from build123d import *

# Parameters (mm, degrees)
SKETCH1_W            = 388.7
SKETCH1_H            = 435.95
SKETCH1_W_2          = 45.6
SKETCH1_H_2          = 430.25
BOSS_EXTRUDE1_DEPTH  = 189
BOSS_EXTRUDE2_START  = -433.45
SKETCH2_W            = 388.7
SKETCH2_H            = 3.2
BOSS_EXTRUDE2_DEPTH  = 430.25
CUT_EXTRUDE1_DEPTH   = 25
BOSS_EXTRUDE4_DEPTH  = 3.2
BOSS_EXTRUDE5_DEPTH  = 3.2
BOSS_EXTRUDE6_REACH  = 791.664
CUT_EXTRUDE2_REACH   = 793.231
SKETCH11_W           = 52.59
SKETCH11_H           = 168.019571709
BOSS_EXTRUDE7_DEPTH  = 3.2
BOSS_EXTRUDE8_DEPTH  = 3.2
SKETCH14_W           = 388.7
SKETCH14_H           = 3.2
BOSS_EXTRUDE9_DEPTH  = 40
SKETCH15_W           = 388.7
SKETCH15_H           = 3.2
BOSS_EXTRUDE10_DEPTH = 40
SKETCH16_W           = 693.36
SKETCH16_H           = 3.2
BOSS_EXTRUDE11_DEPTH = 43.15
SKETCH17_W           = 693.36
SKETCH17_H           = 3.2
BOSS_EXTRUDE12_DEPTH = 43.15
BOSS_EXTRUDE13_DEPTH = 388.7


with BuildPart() as part:
    # Sketch1 → Boss-Extrude1 (new body)
    with BuildSketch(Plane(origin=(0, 0, 0), x_dir=(1, 0, 0), z_dir=(0, 1, 0))):
        with Locations((191.15, 214.775)):
            Rectangle(SKETCH1_W, SKETCH1_H)
        with Locations((22.8, 215.125)):
            Rectangle(SKETCH1_W_2, SKETCH1_H_2, mode=Mode.SUBTRACT)
        with Locations((359.5, 215.125)):
            Rectangle(SKETCH1_W_2, SKETCH1_H_2, mode=Mode.SUBTRACT)
        with Locations((70.9, 215.125)):
            Rectangle(SKETCH1_W_2, SKETCH1_H_2, mode=Mode.SUBTRACT)
        with Locations((119, 215.125)):
            Rectangle(SKETCH1_W_2, SKETCH1_H_2, mode=Mode.SUBTRACT)
        with Locations((167.1, 215.125)):
            Rectangle(SKETCH1_W_2, SKETCH1_H_2, mode=Mode.SUBTRACT)
        with Locations((215.2, 215.125)):
            Rectangle(SKETCH1_W_2, SKETCH1_H_2, mode=Mode.SUBTRACT)
        with Locations((263.3, 215.125)):
            Rectangle(SKETCH1_W_2, SKETCH1_H_2, mode=Mode.SUBTRACT)
        with Locations((311.4, 215.125)):
            Rectangle(SKETCH1_W_2, SKETCH1_H_2, mode=Mode.SUBTRACT)
    extrude(amount=BOSS_EXTRUDE1_DEPTH)

    # Sketch2 → Boss-Extrude2 (add)
    with BuildSketch(Plane.XY.offset(3.2).offset(BOSS_EXTRUDE2_START)):
        with Locations((191.15, 1.6)):
            Rectangle(SKETCH2_W, SKETCH2_H)
    extrude(amount=BOSS_EXTRUDE2_DEPTH)

    # Sketch3 → Cut-Extrude1 (cut)
    with BuildSketch(Plane(origin=(0, 189, 0), x_dir=(1, 0, 0), z_dir=(0, 1, 0))):
        Polygon((0, 430.25), (0, 432.75), (382.3, 432.75), (382.3, 430.25), (336.7, 430.25), (336.7, 0), (334.2, 0), (334.2, 430.25), (288.6, 430.25), (288.6, 0), (286.1, 0), (286.1, 430.25), (240.5, 430.25), (240.5, 0), (238, 0), (238, 430.25), (192.4, 430.25), (192.4, 0), (189.9, 0), (189.9, 430.25), (144.3, 430.25), (144.3, 0), (141.8, 0), (141.8, 430.25), (96.2, 430.25), (96.2, 0), (93.7, 0), (93.7, 430.25), (48.1, 430.25), (48.1, 0), (45.6, 0), (45.6, 430.25), align=None)
    extrude(amount=-CUT_EXTRUDE1_DEPTH, mode=Mode.SUBTRACT)

    # Sketch4 → Boss-Extrude4 (add)
    with BuildSketch(Plane(origin=(385.5, 0, 0), x_dir=(0, 0, -1), z_dir=(1, 0, 0))):
        Polygon((432.75, 189), (662.75, 0), (432.75, 0), align=None)
    extrude(amount=-BOSS_EXTRUDE4_DEPTH)

    # Sketch7 → Boss-Extrude5 (add)
    with BuildSketch(Plane.ZY.offset(3.2)):
        Polygon((-432.75, 164), (-432.75, 189), (-662.75, 0), (-432.75, 0), align=None)
    extrude(amount=-BOSS_EXTRUDE5_DEPTH)

    # Sketch9 → Boss-Extrude6 (add, up to next)
    with BuildSketch(Plane(origin=(0, 0, 0), x_dir=(0, 0, -1), z_dir=(1, 0, 0)), mode=Mode.PRIVATE) as boss_extrude6_sk1:
        Polygon((662.75, 0), (658.855820106, 3.2), (432.75, 3.2), (432.75, 0), align=None)
    boss_extrude6_tool1 = extrude(boss_extrude6_sk1.sketch, amount=BOSS_EXTRUDE6_REACH, mode=Mode.PRIVATE) - part.part
    add(boss_extrude6_tool1.solids().sort_by_distance((0, 1.595446, -546.779226))[0])

    # Sketch11 → Cut-Extrude2 (cut, up to next)
    with BuildSketch(Plane(origin=(385.5, 0, 0), x_dir=(0, 0, -1), z_dir=(1, 0, 0)), mode=Mode.PRIVATE) as cut_extrude2_sk1:
        with Locations((636.455, 84.009785855)):
            Rectangle(SKETCH11_W, SKETCH11_H)
    cut_extrude2_tool1 = extrude(cut_extrude2_sk1.sketch, amount=-CUT_EXTRUDE2_REACH, mode=Mode.PRIVATE) & part.part
    add(cut_extrude2_tool1.solids().sort_by_distance((385.5, 84.009786, -636.455))[0], mode=Mode.SUBTRACT)

    # Sketch12 → Boss-Extrude7 (add)
    with BuildSketch(Plane(origin=(385.5, 0, 0), x_dir=(0, 0, -1), z_dir=(1, 0, 0))):
        Polygon((456.376412276, 189), (610.16, 62.630008348), (610.16, 43.21526087), (432.75, 189), align=None)
    extrude(amount=-BOSS_EXTRUDE7_DEPTH)

    # Sketch13 → Boss-Extrude8 (add)
    with BuildSketch(Plane.ZY.offset(3.2)):
        Polygon((-610.16, 62.630008348), (-610.16, 43.21526087), (-432.75, 189), (-456.376412276, 189), align=None)
    extrude(amount=-BOSS_EXTRUDE8_DEPTH)

    # Sketch14 → Boss-Extrude9 (add)
    with BuildSketch(Plane(origin=(0, 0, -610.16), x_dir=(-1, 0, 0), z_dir=(0, 0, -1))):
        with Locations((-191.15, 1.6)):
            Rectangle(SKETCH14_W, SKETCH14_H)
    extrude(amount=BOSS_EXTRUDE9_DEPTH)

    # Sketch15 → Boss-Extrude10 (add)
    with BuildSketch(Plane.XY.offset(3.2)):
        with Locations((191.15, 1.6)):
            Rectangle(SKETCH15_W, SKETCH15_H)
    extrude(amount=BOSS_EXTRUDE10_DEPTH)

    # Sketch16 → Boss-Extrude11 (add)
    with BuildSketch(Plane(origin=(385.5, 0, 0), x_dir=(0, 0, -1), z_dir=(1, 0, 0))):
        with Locations((303.48, 1.6)):
            Rectangle(SKETCH16_W, SKETCH16_H)
    extrude(amount=BOSS_EXTRUDE11_DEPTH)

    # Sketch17 → Boss-Extrude12 (add)
    with BuildSketch(Plane.ZY.offset(3.2)):
        with Locations((-303.48, 1.6)):
            Rectangle(SKETCH17_W, SKETCH17_H)
    extrude(amount=BOSS_EXTRUDE12_DEPTH)

    # Sketch18 → Boss-Extrude13 (add)
    with BuildSketch(Plane.ZY.offset(3.2)):
        Polygon((-457.200187026, 191.3), (3.2, 191.3), (3.2, 189), (-456.376412276, 189), (-610.16, 62.630008348), (-610.16, 3.2), (-612.46, 3.2), (-612.46, 63.716936295), align=None)
    extrude(amount=-BOSS_EXTRUDE13_DEPTH)


solid = part.part
For this review, take the finished solid that the model builds, in its own axes (mm). A direction names the side the tool comes from. Give positions to 0.01 mm unless a question says otherwise; leave off trailing zeros. Loops run counter-clockwise (first coordinate to the right, second up) from the corner with the lowest first, then second, coordinate; pieces in that order, holes last.
Item 1: Tool access review of faces 1 (the flat face through (-3.2, 99, -300)), 2 (the flat face through (288.6, 82, -212)): name each direction out of +Z, -Z, +X, -X, +Y, -Y from which nothing blocks a thin tool from reaching the whole face with its end or side.
Item 2: For line 1 along Z through (x, y) = (90, 17); line 2 along Y through (x, z) = (82, -298.5); line 3 along Z through (x, y) = (326, 132.5), list the stretches that pass through material, from the lowest coordinate up.
Item 3: Draft analysis for pull direction X (two halves, no side actions). For faces 3 (the flat face through (385.5, 99, -300)), 4 (the flat face through (188, 99, 3.2)), 5 (the flat face through (188.47, 126.7, -532.19)), 6 (the flat face through (359, 82, -430.25)), state which applies: +X half, -X half, draft (parallel to the pull), parting line (faces both ways), or undercut.
Item 4: Take a section at B-B, the plane z = -531.5. State the section outline as (x, y) points, and give its area (3 significant figures).
Item 5: Take a section at C-C, the plane y = 31. Give the number of separate pieces and of enclosed holes in the cut face, and give its area (3 significant figures).
Item 6: Insertion check: pin 1 (1 mm diameter, centred on y = 67.5, z = -159.5, fed in from -X); pin 2 (2 mm diameter, centred on x = 285.5, y = 30, fed in from +Z); pin 3 (6 mm diameter, centred on y = 132, z = -139, fed in from +X). Each pin has a flat end and moves straight along its axis. Give the tip position at first contact, or say it passes through.
Item 7: Take a section at A-A, the plane x = 173. State the section outline as (y, z) points, and give its area (3 significant figures).
Calculated:
1. face 1: +Z, -Z, -X, +Y
1. face 2: none
2. line 1: z = -612.46 to -610.16, -432.75 to -430.25, 0 to 3.2
2. line 2: y = 0 to 3.2, 189 to 191.3
2. line 3: z = -528.76 to -525.13, -432.75 to -430.25, 0 to 3.2
3. face 3: +X half
3. face 4: draft
3. face 5: undercut
3. face 6: undercut
4. outline: (-46.35, 0) - (428.65, 0) - (428.65, 3.2) - (385.5, 3.2) - (385.5, 130.24) - (-3.2, 130.24) - (-3.2, 3.2) - (-46.35, 3.2) - close; hole (0, 3.2) - (382.3, 3.2) - (382.3, 127.27) - (0, 127.27) - close
4. area: 3,470 mm2
5. separate pieces: 1
5. enclosed holes: 9
5. area: 14,500 mm2
6. pin 1: stops at x = -3.2
6. pin 2: stops at z = 3.2
6. pin 3: stops at x = 385.5
7. outline: (0, -650.16) - (3.2, -650.16) - (3.2, -612.46) - (63.72, -612.46) - (191.3, -457.2) - (191.3, 3.2) - (3.2, 3.2) - (3.2, 43.2) - (0, 43.2) - close; hole (3.2, -610.16) - (62.63, -610.16) - (189, -456.38) - (189, 0) - (3.2, 0) - (3.2, -430.25) - (164, -430.25) - (164, -432.75) - (3.2, -432.75) - close
7. area: 4,870 mm2
